Source: CAD feature listing. Evaluate the final solid. Frame: model axes, mm. Face numbers are marked on the shaded views. A direction names the side the tool comes from. Give positions to 0.01 mm unless a question says otherwise; leave off trailing zeros. Write each loop counter-clockwise with the first axis right and the second up, starting at its lowest first coordinate (ties: lowest second). Pieces come first, ordered by that corner, then holes. Notation, with made-up numbers: M 33,-5 L 65,-5 A19 cw 65,20 Z; hole C 63.5,85 d2. An arc over 180 degrees is marked long. Use CSV: the item, a comma, the result in double quotes. Start each with the question number.
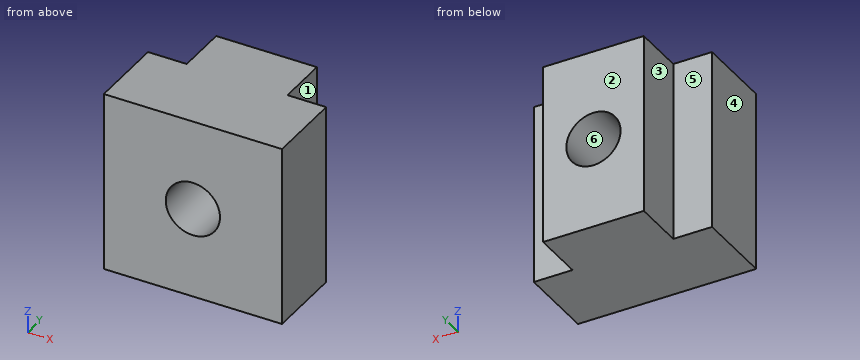
from build123d import *

# Parameters (mm, degrees)
ESQUISSE1_W             = 13.8
ESQUISSE1_H             = 6
BOSS_EXTRU_1_DEPTH      = 14
ESQUISSE2_W             = 7.8
ESQUISSE2_H             = 4
BOSS_EXTRU_2_DEPTH      = 14
ESQUISSE3_R             = 2.1
ENL_V_MAT_EXTRU_1_DEPTH = 23.05538483


with BuildPart() as part:
    # Esquisse1 → Boss.-Extru.1 (new body)
    with BuildSketch(Plane.XY):
        with Locations((6.9, 3)):
            Rectangle(ESQUISSE1_W, ESQUISSE1_H)
    extrude(amount=BOSS_EXTRU_1_DEPTH)

    # Esquisse2 → Boss.-Extru.2 (add)
    with BuildSketch(Plane.XY.offset(14)):
        with Locations((6.9, 8)):
            Rectangle(ESQUISSE2_W, ESQUISSE2_H)
    extrude(amount=-BOSS_EXTRU_2_DEPTH)

    # Esquisse3 → Enlèv. mat.-Extru.1 (cut, through all)
    with BuildSketch(Plane(origin=(0, 10, 0), x_dir=(1, 0, 0), z_dir=(0, 1, 0))):
        with Locations(Location((6.9, -7, 0), (0, 0, 180))):
            Circle(ESQUISSE3_R)
    extrude(amount=-ENL_V_MAT_EXTRU_1_DEPTH, mode=Mode.SUBTRACT)


solid = part.part
1. Section C-C on z = 3. Return loops of the section in (x, y), then the cut area to 3 significant figures.
2. Access query for the marked faces 1, 2 and 3. Directions: +Z, -Z, +X, -X, +Y, -Y. A direction counts if a zero-diameter tool reaches every point of the face in a straight line with its end or side. Return the directions, or none.
3. Section D-D on y = 8.25. Return loops of the section in (x, z), then the cut area to 3 significant figures.
4. Section A-A on z = 7. Return loops of the section in (x, y).
5. Line query: probe 1 along Z at (x, y) = (6.9, 2.75); probe 2 along Y at (x, z) = (11.25, 8.25); probe 3 along X at (y, z) = (4.25, 6.5). Output: solid intervals per line, ascending.
6. First-contact query: pin 1 (1 mm diameter, centred on y = 4.5, z = 10.5, fed in from -X); pin 2 (2.5 mm diameter, centred on x = 1, z = 9.5, fed in from +Y); pin 3 (1.2 mm diameter, centred on y = 8, z = 9, fed in from +X). Flat tips, straight axial feed; report the tip coordinate or a pass-through.
7. Pull-direction query (X, two-part tool) for the marked faces 4, 5 and 6; classes: released by +X, released by -X, zero draft, split by the parting line, or undercut.
8. Section B-B on x = 6.9. Return loops of the section in (y, z), then the cut area to 3 significant figures.
Resolved:
1,outline,"M 0,0 L 13.8,0 L 13.8,6 L 10.8,6 L 10.8,10 L 3,10 L 3,6 L 0,6 Z"
1,area,"114 mm2"
2,face 1,"+Z, -Z, +X, +Y"
2,face 2,"+Z, -Z, +X, -X, +Y"
2,face 3,"+Z, -Z, -X, +Y"
3,outline,"M 3,0 L 10.8,0 L 10.8,14 L 3,14 Z; hole C 6.9,7 d4.2"
3,area,"95.3 mm2"
4,outline,"M 0,0 L 4.8,0 L 4.8,10 L 3,10 L 3,6 L 0,6 Z; M 9,0 L 13.8,0 L 13.8,6 L 10.8,6 L 10.8,10 L 9,10 Z"
5,probe 1,"z = 0 to 4.9, 9.1 to 14"
5,probe 2,"y = 0 to 6"
5,probe 3,"x = 0 to 4.86, 8.94 to 13.8"
6,pin 1,"stops at x = 0"
6,pin 2,"stops at y = 6"
6,pin 3,"stops at x = 10.8"
7,face 4,"released by -X"
7,face 5,"zero draft"
7,face 6,"undercut"
8,outline,"M 0,0 L 10,0 L 10,4.9 L 0,4.9 Z; M 0,9.1 L 10,9.1 L 10,14 L 0,14 Z"
8,area,"98.0 mm2"
